Answer from the drawing. Dimensions are ordinates in mm from the lowest x, y and z of the part. A direction names the side the tool comes from. Round coordinates to 2 decimals unless told otherwise and drop trailing zeros. Order: outer loops, then holes, each group sorted by start corner. A loop starts at its lowest first (then second) coordinate and runs counter-clockwise, first axis right, second up.
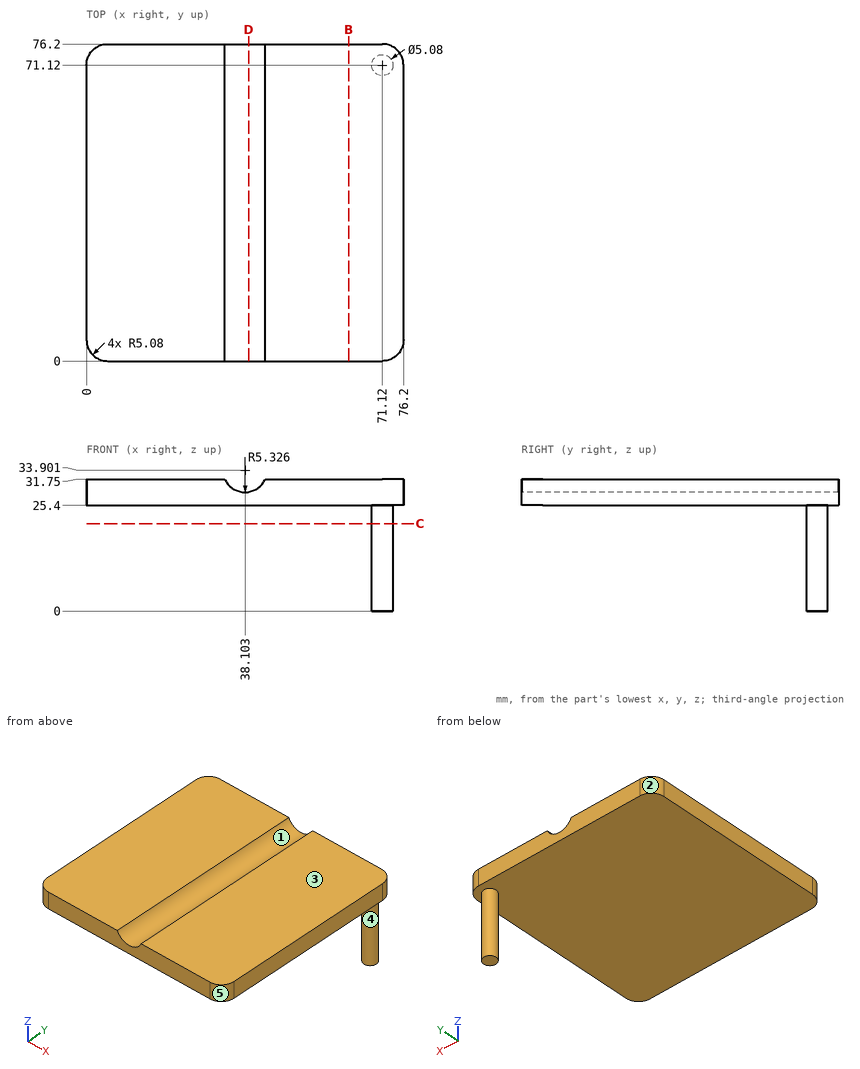
Q1. For the marked faces 4 and 5, determine the directions among +Z, -Z, +X, -X, +Y, -Y from which every point of the face is accessible in a straight line to the end or side of a thin tool.
Outcome:
face 4: -Z
face 5: +Z, -Z, +X, -Y
Q2. A cutting plane is placed at B-B, the plane x = 63. Give the vertices of the cut face in (y, z), plus the area to 3 significant figures.
Outcome:
outline: (0, 25.4) - (76.2, 25.4) - (76.2, 31.75) - (0, 31.75) - close
area: 484 mm2
Q3. For a pull along X with two mould halves and no side action, classify the marked faces 1, 2 and 3 as released by +X, released by -X, zero draft, split by the parting line, or undercut.
Outcome:
face 1: undercut
face 2: released by -X
face 3: zero draft
Q4. A cutting plane is placed at D-D, the plane x = 39. Give the vertices of the cut face in (y, z), plus the area to 3 significant figures.
Outcome:
outline: (0, 25.4) - (76.2, 25.4) - (76.2, 28.65) - (0, 28.65) - close
area: 248 mm2
Q5. A cutting plane is placed at C-C, the plane z = 21. Give the vertices of the cut face in (x, y).
Outcome:
outline: circle Ø5.08 at (71.12, 71.12)
Q6. Straight lines are drawn through the part: probe 1 along Z at (x, y) = (19.5, 45.5); probe 2 along Y at (x, z) = (71, 3); probe 3 along X at (y, z) = (54, 29) (1 decimal). For each, find the intervals that lie inside material, in ascending order.
Outcome:
probe 1: z = 25.4 to 31.75
probe 2: y = 68.58 to 73.66
probe 3: x = 0 to 36, 40.2 to 76.2
Q7. Flat-ended cylindrical pins translate along their axes: pin 1 (1 mm diameter, centred on y = 58, z = 24, fed in from -X); pin 2 (5 mm diameter, centred on x = 20.5, y = 40.5, fed in from -Z). Find the tip coordinate at first contact, or state that the pin passes through.
Outcome:
pin 1: passes through
pin 2: stops at z = 25.4
